Verification items for this drawing (mm, ordinates from the low corner). A direction names the side the tool comes from. Round coordinates to 2 decimals unless told otherwise and drop trailing zeros. Write each loop counter-clockwise with the first axis right and the second up, starting at its lowest first coordinate (ties: lowest second). Pieces come first, ordered by that corner, then holes.
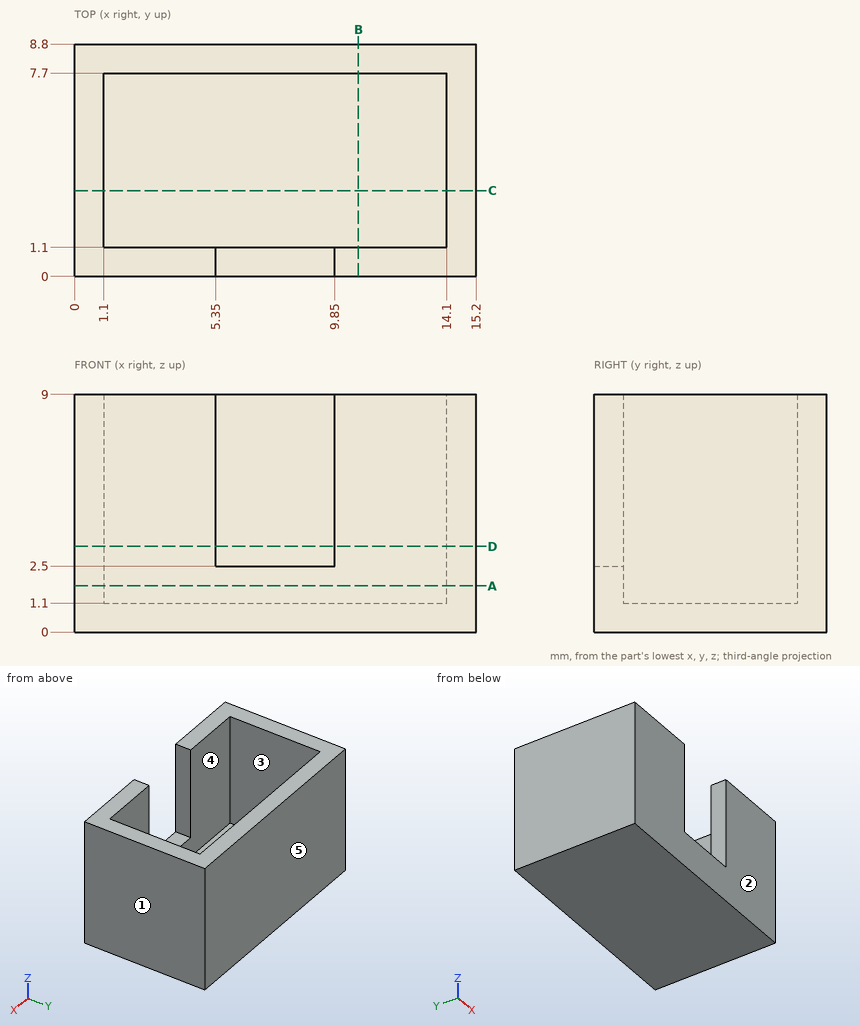
1. Access from +Z, -Z, +X, -X, +Y, -Y to the whole of each face (thin tool, end or side, straight path). Record for the marked faces 4 and 5.
2. Section check D-D (z = 3.25). Record the cut outline in (x, y).
3. Section check C-C (y = 3.25). Record the cut outline in (x, z), plus the area to 3 significant figures.
4. Section check B-B (x = 10.75). Record the cut outline in (y, z).
5. Section check A-A (z = 1.75). Record the cut outline in (x, y).
6. Release check for a two-part mould opening along Y. For the marked faces 1, 2 and 3 record: +Y half, -Y half, draft (parallel to the pull), parting line (faces both ways), or undercut.
7. Scan lines: line 1 along X through (y, z) = (5, 8); line 2 along Y through (x, z) = (4.5, 7.5); line 3 along Z through (x, y) = (2, 2.5). Record each from-to range of solid material in increasing order.
8. Depth check by flat-ended pin: pin 1 Ø1.2 at (x, y) = (7, 0.5) entering from +Z; pin 2 Ø1 at (x, y) = (13, 3.5) entering from +Z. Enter the tip coordinate at first touch or a pass-through.
Results below:
1. face 4: +Z
1. face 5: +Z, -Z, +X, -X, +Y
2. outline: (0, 0) - (5.35, 0) - (5.35, 1.1) - (1.1, 1.1) - (1.1, 7.7) - (14.1, 7.7) - (14.1, 1.1) - (9.85, 1.1) - (9.85, 0) - (15.2, 0) - (15.2, 8.8) - (0, 8.8) - close
3. outline: (0, 0) - (15.2, 0) - (15.2, 9) - (14.1, 9) - (14.1, 1.1) - (1.1, 1.1) - (1.1, 9) - (0, 9) - close
3. area: 34.1 mm2
4. outline: (0, 0) - (8.8, 0) - (8.8, 9) - (7.7, 9) - (7.7, 1.1) - (1.1, 1.1) - (1.1, 9) - (0, 9) - close
5. outline: (0, 0) - (15.2, 0) - (15.2, 8.8) - (0, 8.8) - close; hole (1.1, 1.1) - (14.1, 1.1) - (14.1, 7.7) - (1.1, 7.7) - close
6. face 1: draft
6. face 2: -Y half
6. face 3: undercut
7. line 1: x = 0 to 1.1, 14.1 to 15.2
7. line 2: y = 0 to 1.1, 7.7 to 8.8
7. line 3: z = 0 to 1.1
8. pin 1: stops at z = 2.5
8. pin 2: stops at z = 1.1
